Read the model definition and answer for the solid it produces. Units are mm, in the model's axes. A direction names the side the tool comes from. Give positions to 0.01 mm unless a question says otherwise; leave off trailing zeros. Order: outer loops, then holes, each group sorted by start corner. A loop starts at its lowest first (then second) coordinate and runs counter-clockwise, first axis right, second up. Notation, with made-up numbers: (52.25, -34) -> (109.25, -34) arc R9 cw to (109.25, -21) -> close; hole circle Ø7 at (56.5, 25). An arc over 180 degrees is marked (long way). Use one line per item in the form item = value.
```python
from build123d import *

# Parameters (mm, degrees)
F1_DEPTH       = 12.5
F2_R           = 2.5
F3_DEPTH       = 25
F5_D           = 5
F5_DEPTH       = 12
F5_CBORE_D     = 5
F5_CBORE_DEPTH = 5
F6_R           = 5
F7_R           = 5
F8_R           = 1.190337


with BuildPart() as f1:
    # F0 (on Front) → F1 (new body, symmetric)
    with BuildSketch(Plane.XZ):
        with BuildLine():
            Line((-10.22166, 0), (39.715874, 0))
            Line((39.715874, 0), (39.715874, 1.9))
            Line((39.715874, 1.9), (-10.284126, 1.9))
            ThreePointArc((-10.284126, 1.9), (-18.558483, 6.686742), (-18.533697, 16.245888))
            Line((-18.533697, 16.245888), (-1.153674, 33.625912))
            Line((-1.153674, 33.625912), (-2.497177, 34.969415))
            Line((-2.497177, 34.969415), (-20.174846, 17.291745))
            ThreePointArc((-20.174846, 17.291745), (-20.19751, 5.768283), (-10.22166, 0))
        make_face()
    extrude(amount=F1_DEPTH, both=True)

    # F2 (on face) → F3 (cut)
    with BuildSketch(Plane.XY.offset(1.9)):
        with Locations((4.715874, 0)):
            Circle(F2_R)
        with BuildLine():
            Line((35.217137, 2.606625), (20.217137, 2.606625))
            ThreePointArc((20.217137, 2.606625), (17.717137, 0.106625), (20.217137, -2.393375))
            Line((20.217137, -2.393375), (35.217137, -2.393375))
            ThreePointArc((35.217137, -2.393375), (37.717137, 0.106625), (35.217137, 2.606625))
        make_face()
    extrude(amount=-F3_DEPTH, mode=Mode.SUBTRACT)

    # F5
    with Locations(Plane(origin=(-18.733296, 0, 18.733296), x_dir=(0, -1, 0), z_dir=(-0.707107, 0, 0.707107))):
        with Locations((-5, 17.293558), (5, 17.293558)):
            CounterBoreHole(F5_D / 2, F5_CBORE_D / 2, F5_CBORE_DEPTH, depth=F5_DEPTH)

    # F6
    f6_edges = [f1.edges().sort_by_distance(p)[0] for p in [
        (39.715874, -12.5, 0.95),
        (39.715874, 12.5, 0.95),
    ]]
    fillet(f6_edges, radius=F6_R)

    # F7
    f7_edges = [f1.edges().sort_by_distance(p)[0] for p in [
        (-1.825425, -12.5, 34.297663),
        (-1.825425, 12.5, 34.297663),
    ]]
    fillet(f7_edges, radius=F7_R)

    # F8
    f8_edges = [f1.edges().sort_by_distance(p)[0] for p in [
        (-18.533697, 0, 16.245888),
        (-10.284126, 0, 1.9),
    ]]
    fillet(f8_edges, radius=F8_R)


solid = f1.part
```
Item 1: The part is cut by section A-A on y = -3.5. Give the vertices of the cut face in (x, z), and give its area (3 significant figures).
Checks:
outline = (-20.17, 17.29) arc R11.51 ccw to (-10.22, 0) -> (39.72, 0) -> (39.72, 1.9) -> (-10.28, 1.9) arc R9.54 cw to (-18.62, 16.1) arc R1.19 cw to (-18.42, 16.36) -> (-6.58, 28.2) -> (-7.92, 29.55) -> close; (-5.09, 32.38) -> (-3.75, 31.03) -> (-1.15, 33.63) -> (-2.5, 34.97) -> close
area = 176 mm²
Item 2: Determine the mould class of faces 1 (the cylindrical face through (38.212, -11.074, 0.963)), 2 (the flat face through (14, 0, 0)), 3 (the cylindrical face through (37.717, 0.052, 0.963)) for opening direction X: +X half, -X half, draft (parallel to the pull), parting line (faces both ways), or undercut.
Checks:
face_1 = +X half
face_2 = draft
face_3 = undercut
Item 3: Straight lines are drawn through the part: L1, parallel to Z at x = 35.5, y = 9; L2, parallel to Z at x = -12, y = 5.5; L3, parallel to Z at x = -15, y = 0.75. For each, find the intervals that lie inside material, in ascending order. Write a range as from..to.
Checks:
L1 = 0..1.9
L2 = 0.14..2.06, 22.78..25.47
L3 = 1.04..3.15, 19.78..22.47
Item 4: Which of the six approach directions +Z, -Z, +X, -X, +Y, -Y give full straight-line access (tool end or side, diameter ignored) to faces 4 (the cylindrical face through (-2.898, -11.074, 33.244)), 5 (the flat face through (-9.91, -0.18, 24.87)), 6 (the flat face through (28, -2.393, 1))?
Checks:
face_4 = +Z, +X, -Y
face_5 = +X, +Y, -Y
face_6 = +Z, -Z
Item 5: The part is cut by section D-D on z = 7. Give the vertices of the cut face in (x, y), and give its area (3 significant figures).
Checks:
outline = (-20.81, -12.5) -> (-18.73, -12.5) -> (-18.73, 12.5) -> (-20.81, 12.5) -> close
area = 52.0 mm²
Item 6: The part is cut by section C-C on x = -12.5. Give the vertices of the cut face in (y, z).
Checks:
outline = (-12.5, 0.23) -> (12.5, 0.23) -> (12.5, 2.16) -> (-12.5, 2.16) -> close; (-12.5, 22.28) -> (12.5, 22.28) -> (12.5, 24.97) -> (-12.5, 24.97) -> close
Item 7: The part is cut by section B-B on y = 1.5. Give the vertices of the cut face in (x, z), and give its area (3 significant figures).
Checks:
outline = (-20.17, 17.29) arc R11.51 ccw to (-10.22, 0) -> (2.72, 0) -> (2.72, 1.9) -> (-10.28, 1.9) arc R9.54 cw to (-18.62, 16.1) arc R1.19 cw to (-18.42, 16.36) -> (-1.15, 33.63) -> (-2.5, 34.97) -> close; (6.72, 0) -> (18.14, 0) -> (18.14, 1.9) -> (6.72, 1.9) -> close; (37.29, 0) -> (39.72, 0) -> (39.72, 1.9) -> (37.29, 1.9) -> close
area = 140 mm²
Item 8: Given pin 1 Ø8 at (y, z) = (6, 28) entering from -X; pin 2 Ø8 at (x, y) = (4.72, 0) entering from +Z; pin 3 Ø2 at (y, z) = (4, 7.5) entering from -X; pin 4 Ø6 at (x, z) = (25.5, 5.5) entering from +Y, each flat-ended and moving along its own axis, determine where each tip first touches the part or whether it passes through.
Checks:
pin_1 = -13.47
pin_2 = 1.9
pin_3 = -21.33
pin_4 = through
